Can you work these out from the model? Positions are in its coordinate system, mm. Round coordinates to 2 decimals unless told otherwise and drop trailing zeros. Loops run counter-clockwise (first coordinate to the right, second up) from the corner with the lowest first, then second, coordinate; pieces in that order, holes last. Notation, with made-up numbers: M -23,3.5 L 19,3.5 A24 ccw 19,38.5 Z; hole C -14.5,-21 d6. An arc over 180 degrees is marked long. Use a Markdown table: item, result. Add a question column.
Autodesk Inventor part; units mm, degrees
ref_plane "YZ Plane" through (0, 0, 0) normal (1, 0, 0) x (0, 1, 0)
ref_plane "XZ Plane" through (0, 0, 0) normal (0, 1, 0) x (-1, 0, 0)
ref_plane "XY Plane" through (0, 0, 0) normal (0, 0, 1) x (1, 0, 0)
sketch "Sketch2" plane through (0, 0, 0) normal (0, 0, 1) x (1, 0, 0)
  circle A0 centre (175, 88) radius 3.2
  circle A1 centre (175, -118) radius 3.2
  circle A2 centre (-175, -118) radius 3.2
  circle A3 centre (-175, 88) radius 3.2
  line L0 (-185, 98) -> (185, 98)
  line L1 (185, 98) -> (185, -128)
  line L2 (185, -128) -> (-185, -128)
  line L3 (-185, -128) -> (-185, 98)
  line L4 (-121, -108) -> (-81, -108)
  line L5 (-81, -108) -> (-81, -118.5)
  line L6 (-81, -118.5) -> (-121, -118.5)
  line L7 (-121, -118.5) -> (-121, -108)
  line L8 (-61, -108) -> (-21, -108)
  line L9 (-21, -108) -> (-21, -118.5)
  line L10 (-21, -118.5) -> (-61, -118.5)
  line L11 (-61, -118.5) -> (-61, -108)
  line L12 (21, -108) -> (61, -108)
  line L13 (61, -108) -> (61, -118.5)
  line L14 (61, -118.5) -> (21, -118.5)
  line L15 (21, -118.5) -> (21, -108)
  line L16 (81, -108) -> (121, -108)
  line L17 (121, -108) -> (121, -118.5)
  line L18 (121, -118.5) -> (81, -118.5)
  line L19 (81, -118.5) -> (81, -108)
  circle A4 centre (0, 0) radius 3.2
extrude "Extrusion2" add sketch "Sketch2" along normal mid plane 2
properties part number "bottom_plate"
(1) Suppose I cut it at B-B on z = 0.05. Count the separate pieces of the cut face and the enclosed holes in it, and give its area (3 significant figures).
(2) Suppose I cut it at A-A on x = -36. List the corners of the cut face in (y, z) for me.
(3) If I drill on probe 1 along Y at (x, z) = (-175, 0.3); probe 2 along Y at (x, z) = (0, -0.2); probe 3 along Y at (x, z) = (91.5, -0.1), over which ranges is the centre line in solid material (lowest first)? Write a range as [from, to].
Results below:
| question | item | result |
|---|---|---|
| 1 | separate pieces | 1 |
| 1 | enclosed holes | 9 |
| 1 | area | 81,800 mm² |
| 2 | outline | M -128,-1 L -118.5,-1 L -118.5,1 L -128,1 Z; M -108,-1 L 98,-1 L 98,1 L -108,1 Z |
| 3 | probe 1 | y = [-128, -121.2], [-114.8, 84.8], [91.2, 98] |
| 3 | probe 2 | y = [-128, -3.2], [3.2, 98] |
| 3 | probe 3 | y = [-128, -118.5], [-108, 98] |
